CAD build for the part. Positions are in the model's coordinates, mm. Round coordinates to 2 decimals unless told otherwise and drop trailing zeros. Order: outer loops, then holes, each group sorted by start corner. A loop starts at its lowest first (then second) coordinate and runs counter-clockwise, first axis right, second up.
```python
from build123d import *

# Parameters (mm, degrees)
SKETCH1_R                       = 61.976
BOSS_EXTRUDE1_DEPTH             = 6.35
F_1_4_0_25_DIAMETER_HOLE1_D     = 6.35
F_1_4_0_25_DIAMETER_HOLE1_DEPTH = 44.958
SKETCH4_R                       = 1.905
CUT_EXTRUDE1_DEPTH              = 7.35


with BuildPart() as part:
    # Sketch1 → Boss-Extrude1 (new body)
    with BuildSketch(Plane(origin=(0, 0, 0), x_dir=(1, 0, 0), z_dir=(0, 1, 0))):
        Circle(SKETCH1_R)
    extrude(amount=BOSS_EXTRUDE1_DEPTH)

    # 1/4 (0.25) Diameter Hole1
    with Locations(Plane(origin=(0, 6.35, 0), x_dir=(1, 0, 0), z_dir=(0, 1, 0))):
        with Locations((0, 44.45), (44.45, 0), (0, -44.45), (-44.45, 0), (0, 0)):
            Hole(F_1_4_0_25_DIAMETER_HOLE1_D / 2, depth=F_1_4_0_25_DIAMETER_HOLE1_DEPTH)

    # Sketch4 → Cut-Extrude1 (cut, through all)
    with BuildSketch(Plane(origin=(0, 6.35, 0), x_dir=(1, 0, 0), z_dir=(0, 1, 0))):
        with Locations((12.7, 0)):
            Circle(SKETCH4_R)
    extrude(amount=-CUT_EXTRUDE1_DEPTH, mode=Mode.SUBTRACT)


solid = part.part
```
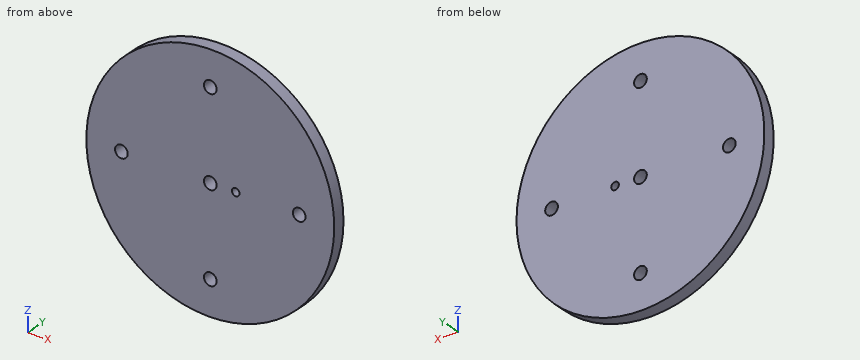
1. Drill centre lines: line 1 (Z direction, x = 0, y = 1.75) (3 decimals); line 2 (X direction, y = 1.75, z = 44.45) (3 decimals); line 3 (X direction, y = 3.25, z = -45). Where is each one in solid material? Low to high.
2. Cut at A-A, the plane z = 0. Write the cut outline in (x, y) (3 decimals).
3. Cut at D-D, the plane z = 44.45. Write the cut outline in (x, y) (3 decimals).
4. Cut at B-B, the plane x = 0. Write the cut outline in (y, z) (3 decimals), and give its area (3 significant figures).
5. Pin check, flat tips, straight feed: P1, Ø1.5, axis at x = -29, y = 3.5, coming from the -Z side; P2, Ø5, axis at x = 44.45, z = 0, coming from the -Y side; P3, Ø5, axis at x = 12.7, z = 0, coming from the -Y side. Stop position of each tip, or through.
6. Cut at C-C, the plane y = 3.25. Write the cut outline in (x, z) (3 decimals), and give its area (3 significant figures).
Outcome:
1. line 1: z = -61.976 to -47.625, -41.275 to -3.175, 3.175 to 41.275, 47.625 to 61.976
1. line 2: x = -43.188 to -3.175, 3.175 to 43.188
1. line 3: x = -42.61 to -3.13, 3.13 to 42.61
2. outline: (-61.976, 0) - (-47.625, 0) - (-47.625, 6.35) - (-61.976, 6.35) - close; (-41.275, 0) - (-3.175, 0) - (-3.175, 6.35) - (-41.275, 6.35) - close; (3.175, 0) - (10.795, 0) - (10.795, 6.35) - (3.175, 6.35) - close; (14.605, 0) - (41.275, 0) - (41.275, 6.35) - (14.605, 6.35) - close; (47.625, 0) - (61.976, 0) - (61.976, 6.35) - (47.625, 6.35) - close
3. outline: (-43.188, 0) - (-3.175, 0) - (-3.175, 6.35) - (-43.188, 6.35) - close; (3.175, 0) - (43.188, 0) - (43.188, 6.35) - (3.175, 6.35) - close
4. outline: (0, -61.976) - (6.35, -61.976) - (6.35, -47.625) - (0, -47.625) - close; (0, -41.275) - (6.35, -41.275) - (6.35, -3.175) - (0, -3.175) - close; (0, 3.175) - (6.35, 3.175) - (6.35, 41.275) - (0, 41.275) - close; (0, 47.625) - (6.35, 47.625) - (6.35, 61.976) - (0, 61.976) - close
4. area: 666 mm2
5. P1: stops at z = -55.16
5. P2: passes through
5. P3: stops at y = 0
6. outline: circle Ø123.952 at (0, 0); hole circle Ø6.35 at (-44.45, 0); hole circle Ø6.35 at (0, -44.45); hole circle Ø6.35 at (0, 0); hole circle Ø6.35 at (0, 44.45); hole circle Ø3.81 at (12.7, 0); hole circle Ø6.35 at (44.45, 0)
6. area: 11,900 mm2
